Design review of the part built by this model. Coordinates are the model's own, in mm. Face numbers are marked on the shaded views. A direction names the side the tool comes from. Round coordinates to 2 decimals unless told otherwise and drop trailing zeros. Write each loop counter-clockwise with the first axis right and the second up, starting at its lowest first coordinate (ties: lowest second). Pieces come first, ordered by that corner, then holes. Notation, with made-up numbers: (-22, 24) -> (14, 24) arc R19 cw to (14, 46) -> close; hole circle Ø9 at (19.5, 70). An arc over 180 degrees is marked (long way). One line per question, with ' | ' between items. Start each with the question number.
1) Insertion check: pin 1 Ø19.5 at (x, y) = (15.5, 209) entering from +Z; pin 2 Ø21.5 at (x, y) = (-3, -5) entering from -Z; pin 3 Ø13.5 at (y, z) = (67, 29) entering from +X; pin 4 Ø5 at (y, z) = (137, 30) entering from -X. Each pin has a flat end and moves straight along its axis. Give the tip position at first contact, or say it passes through.
2) Consider section C-C (z = 8). Give the boundary of the cut face in (x, y).
3) For the marked faces 1, 2 and 3, list the 3-axis set-ups (+Z, -Z, +X, -X, +Y, -Y) from which the entire face can be reached by the end or side of a thin tool; tool diameter is ignored.
4) Consider section D-D (x = 0). Give the boundary of the cut face in (y, z), then the cut area to 3 significant figures.
5) For probe 1 along Y at (x, z) = (-34, 25.5); probe 2 along X at (y, z) = (229, 14); probe 3 along X at (y, z) = (113.5, 22.5), list the stretches that pass through material, from the lowest coordinate up.
6) Consider section B-B (x = 25). Give the boundary of the cut face in (y, z).
7) Consider section A-A (y = 218). Give the boundary of the cut face in (x, z).
8) Mouldability with a two-part tool opening along Y and no side actions: class the marked faces 4, 5, 6 and 7 as +Y half, -Y half, draft (parallel to the pull), parting line (faces both ways), or undercut.
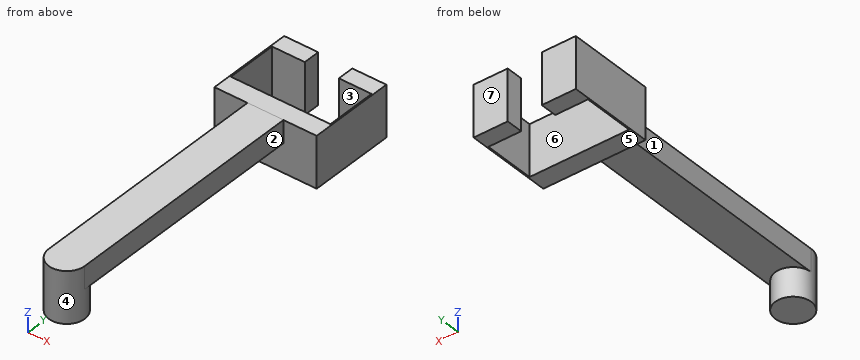
```python
from build123d import *

# Parameters (mm, degrees)
SKETCH2_R           = 13.4112
BOSS_EXTRUDE1_DEPTH = 38.1
SKETCH5_W           = 26.8224
SKETCH5_H           = 184.15
BOSS_EXTRUDE2_DEPTH = 16.7386
SKETCH8_W           = 76.2
SKETCH8_H           = 38.1
BOSS_EXTRUDE3_DEPTH = 13.97
SKETCH9_W           = 1.016
SKETCH9_H           = 38.1
BOSS_EXTRUDE4_DEPTH = 38.1
SKETCH10_W          = 25.4
SKETCH10_H          = 38.1
BOSS_EXTRUDE5_DEPTH = 12.446


with BuildPart() as part:
    # Sketch2 → Boss-Extrude1 (new body)
    with BuildSketch(Plane.XY):
        with Locations(Location((0, 0, 0), (0, 0, 180))):
            Circle(SKETCH2_R)
    extrude(amount=BOSS_EXTRUDE1_DEPTH)

    # Sketch5 → Boss-Extrude2 (add)
    with BuildSketch(Plane.XY.offset(38.1)):
        with Locations((0, 92.075)):
            Rectangle(SKETCH5_W, SKETCH5_H)
    extrude(amount=-BOSS_EXTRUDE2_DEPTH)

    # Sketch8 → Boss-Extrude3 (add)
    with BuildSketch(Plane(origin=(0, 184.15, 0), x_dir=(1, 0, 0), z_dir=(0, 1, 0))):
        with Locations((0, -18.948214994)):
            Rectangle(SKETCH8_W, SKETCH8_H)
    extrude(amount=BOSS_EXTRUDE3_DEPTH)

    # Sketch9 → Boss-Extrude4 (add)
    with BuildSketch(Plane(origin=(0, 198.12, 0), x_dir=(1, 0, 0), z_dir=(0, 1, 0))):
        with Locations((-37.592, -18.948214994)):
            Rectangle(SKETCH9_W, SKETCH9_H)
        with Locations((37.592, -18.948214994)):
            Rectangle(SKETCH9_W, SKETCH9_H)
    extrude(amount=BOSS_EXTRUDE4_DEPTH)

    # Sketch10 → Boss-Extrude5 (add)
    with BuildSketch(Plane(origin=(0, 236.22, 0), x_dir=(1, 0, 0), z_dir=(0, 1, 0))):
        with Locations((-25.4, -18.948214994)):
            Rectangle(SKETCH10_W, SKETCH10_H)
        with Locations((25.4, -18.948214994)):
            Rectangle(SKETCH10_W, SKETCH10_H)
    extrude(amount=BOSS_EXTRUDE5_DEPTH)


solid = part.part
```
From the geometry:
1) pin 1: passes through | pin 2: stops at z = 0 | pin 3: stops at x = 13.41 | pin 4: stops at x = -13.41
2) outline: (-38.1, 184.15) -> (38.1, 184.15) -> (38.1, 248.67) -> (12.7, 248.67) -> (12.7, 236.22) -> (37.08, 236.22) -> (37.08, 198.12) -> (-37.08, 198.12) -> (-37.08, 236.22) -> (-12.7, 236.22) -> (-12.7, 248.67) -> (-38.1, 248.67) -> close; circle Ø26.82 at (0, 0)
3) face 1: +Z, -Z, -X, -Y | face 2: +Z, -Z, +X, -Y | face 3: +Z, -Z
4) outline: (-13.41, 0) -> (13.41, 0) -> (13.41, 21.36) -> (184.15, 21.36) -> (184.15, -0.1) -> (198.12, -0.1) -> (198.12, 38) -> (184.15, 38) -> (184.15, 38.1) -> (-13.41, 38.1) -> close | area: 4,410 mm2
5) probe 1: y = 184.15 to 198.12, 236.22 to 248.67 | probe 2: x = -38.1 to -37.08, 37.08 to 38.1 | probe 3: x = -13.41 to 13.41
6) outline: (184.15, -0.1) -> (198.12, -0.1) -> (198.12, 38) -> (184.15, 38) -> close; (236.22, -0.1) -> (248.67, -0.1) -> (248.67, 38) -> (236.22, 38) -> close
7) outline: (-38.1, -0.1) -> (-37.08, -0.1) -> (-37.08, 38) -> (-38.1, 38) -> close; (37.08, -0.1) -> (38.1, -0.1) -> (38.1, 38) -> (37.08, 38) -> close
8) face 4: undercut | face 5: draft | face 6: undercut | face 7: +Y half
